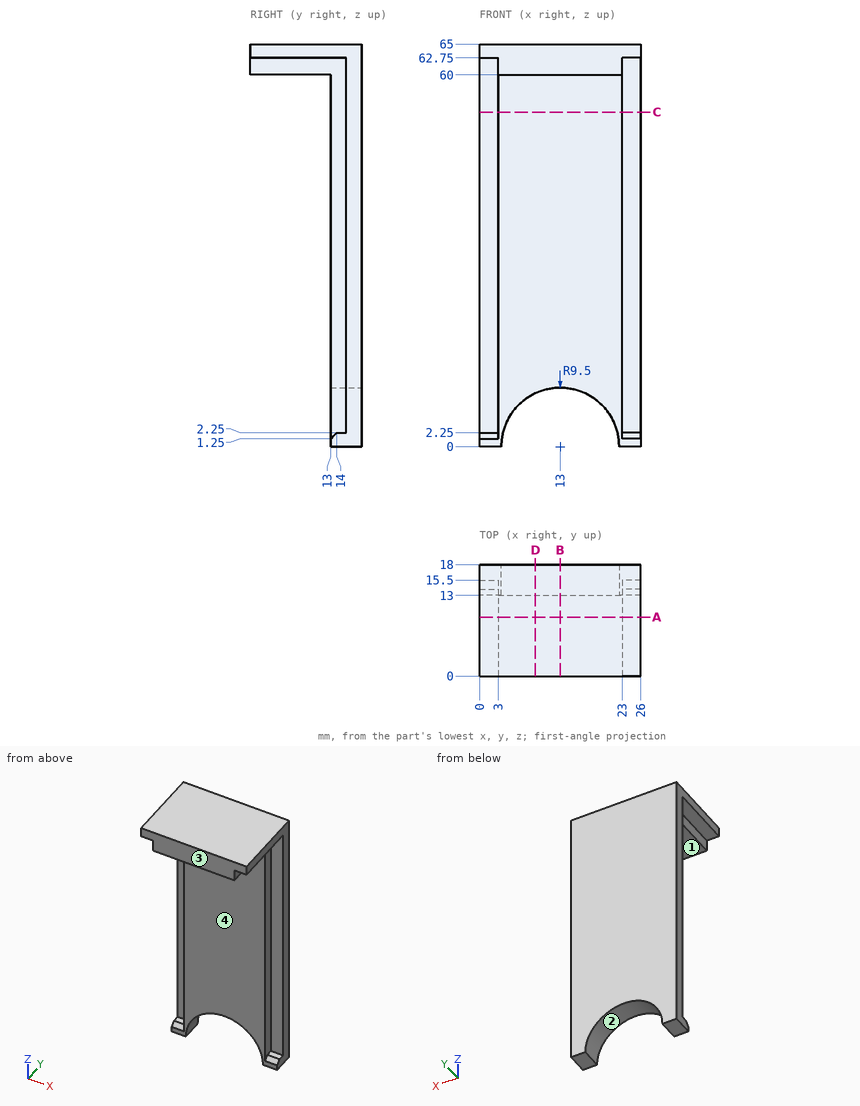
Here's the drawing with two shaded views (mm, measured from the low corner). I have some questions. A direction names the side the tool comes from. Give positions to 0.01 mm unless a question says otherwise; leave off trailing zeros. Loops run counter-clockwise (first coordinate to the right, second up) from the corner with the lowest first, then second, coordinate; pieces in that order, holes last. Notation, with made-up numbers: (20.5, 33) - (71.5, 33) arc R24 ccw to (71.5, 55) - close; hole circle Ø5 at (-24.75, 52.5). An arc over 180 degrees is marked (long way). Answer in a Markdown table with one row per item. Add a question column.
Q1. For pin 1 (5 mm diameter, centred on y = 11, z = 37, fed in from +X); pin 2 (1.5 mm diameter, centred on x = 24.5, z = 30.5, fed in from -Y); pin 3 (6 mm diameter, centred on x = 15, z = 35, fed in from -Y), each with a flat end and sliding along its axis, tell me the tip position at first contact or that it passes through.
Q2. If we section it at C-C (z = 54): List the corners of the cut face in (x, y) for me.
Q3. If we section it at A-A (y = 9.5): List the corners of the cut face in (x, z) for me, plus the area to 4 significant figures.
Q4. If we section it at B-B (x = 13): List the corners of the cut face in (y, z) for me.
Q5. We'd pull the mould along X, two halves only. Please class the marked faces 1 and 2: +X half, -X half, draft (parallel to the pull), parting line (faces both ways), or undercut.
Q6. Which directions (+Z, -Z, +X, -X, +Y, -Y) give clear straight access to the entire face, cutting with the end or side of a thin tool? Please do the marked faces 3 and 4.
Q7. Please list where these lines run through material, in increasing order: L1, parallel to Z at x = 17.5, y = 4; L2, parallel to Y at x = 12.5, z = 44.5; L3, parallel to Z at x = 2.25, y = 8. Write a range as from..to.
Q8. If we section it at D-D (x = 9): List the corners of the cut face in (y, z) for me.
The answers:
| question | item | result |
|---|---|---|
| 1 | pin 1 | stops at x = 23 |
| 1 | pin 2 | stops at y = 15.5 |
| 1 | pin 3 | stops at y = 13 |
| 2 | outline | (0, 15.5) - (3, 15.5) - (3, 13) - (23, 13) - (23, 15.5) - (26, 15.5) - (26, 18) - (0, 18) - close |
| 3 | outline | (0, 62.75) - (3, 62.75) - (3, 60) - (23, 60) - (23, 62.75) - (26, 62.75) - (26, 65) - (0, 65) - close |
| 3 | area | 113.5 mm^2 |
| 4 | outline | (0, 60) - (13, 60) - (13, 9.5) - (18, 9.5) - (18, 65) - (0, 65) - close |
| 5 | face 1 | draft |
| 5 | face 2 | undercut |
| 6 | face 3 | +Z, -Z, +X, -X, -Y |
| 6 | face 4 | -Z, +X, -X, -Y |
| 7 | L1 | z = 60..65 |
| 7 | L2 | y = 13..18 |
| 7 | L3 | z = 62.75..65 |
| 8 | outline | (0, 60) - (13, 60) - (13, 8.62) - (18, 8.62) - (18, 65) - (0, 65) - close |
